Geometry: see drawing. Coordinates: mm, zero at the bounding-box minimum. Coordinates: 2 decimals unless noted, no trailing zeros. Loops run counter-clockwise (first coordinate to the right, second up) from the corner with the lowest first, then second, coordinate; pieces in that order, holes last. Notation, with made-up numbers: (-13.75, -1.75) -> (29.25, -1.75) arc R30 ccw to (29.25, 36.25) -> close; hole circle Ø1 at (-22.5, -38.5). An arc over 180 degrees is marked (long way). Put each result on its own line as item: value. Start each with the question number.
1) Contact query for flat-ended pins moving along their axis: P1, Ø1.5, axis at x = 52.5, z = 1.5, coming from the +Y side; P2, Ø0.9, axis at y = 52.5, z = 1.5, coming from the +X side. Output: stop coordinate, or through.
2) Cut plane C-C (y = 49.5). Return the cut outline in (x, z).
3) Cut plane B-B (x = 49). Return the cut outline in (y, z), plus the area to 3 significant figures.
4) Material intervals for L1, parallel to Y at x = 4.5, z = 2; L2, parallel to Y at x = 10, z = 1.65; L3, parallel to X at y = 48, z = 2.4, sorted ascending.
5) Cut plane A-A (z = 2.5). Return the cut outline in (x, y), plus the area to 3 significant figures.
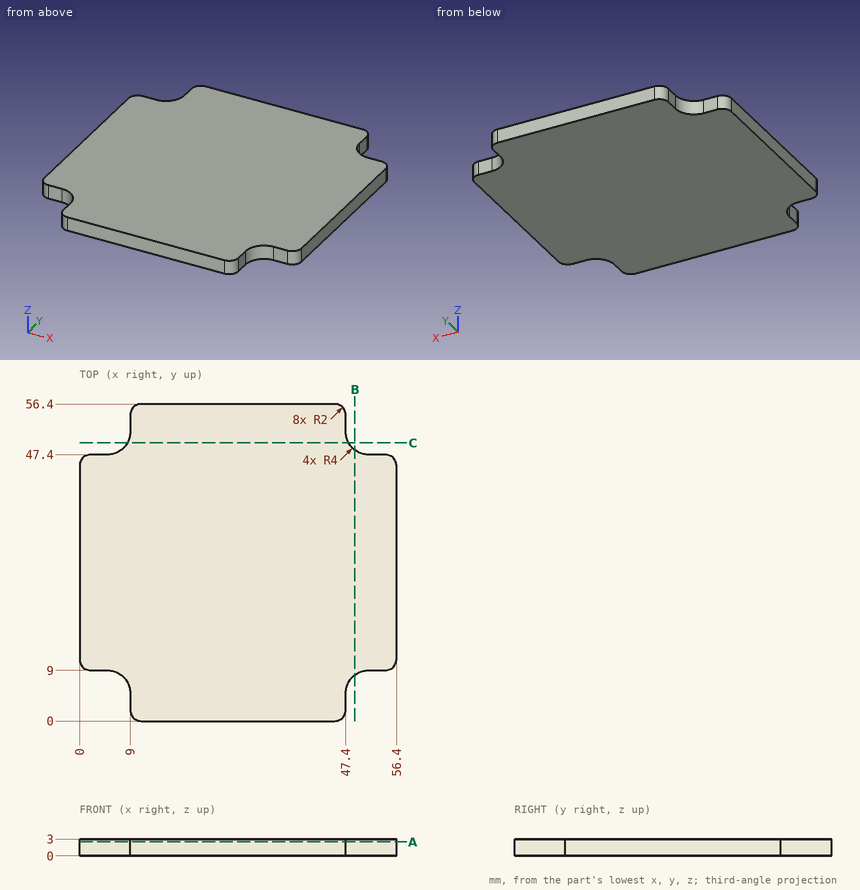
Results found:
1. P1: stops at y = 47.4
1. P2: stops at x = 47.4
2. outline: (8.52, 0) -> (47.88, 0) -> (47.88, 3) -> (8.52, 3) -> close
3. outline: (8.2, 0) -> (48.2, 0) -> (48.2, 3) -> (8.2, 3) -> close
3. area: 120 mm2
4. L1: y = 9 to 47.4
4. L2: y = 0.27 to 56.13
4. L3: x = 7.11 to 49.29
5. outline: (0, 11) arc R2 ccw to (2, 9) -> (5, 9) arc R4 cw to (9, 5) -> (9, 2) arc R2 ccw to (11, 0) -> (45.4, 0) arc R2 ccw to (47.4, 2) -> (47.4, 5) arc R4 cw to (51.4, 9) -> (54.4, 9) arc R2 ccw to (56.4, 11) -> (56.4, 45.4) arc R2 ccw to (54.4, 47.4) -> (51.4, 47.4) arc R4 cw to (47.4, 51.4) -> (47.4, 54.4) arc R2 ccw to (45.4, 56.4) -> (11, 56.4) arc R2 ccw to (9, 54.4) -> (9, 51.4) arc R4 cw to (5, 47.4) -> (2, 47.4) arc R2 ccw to (0, 45.4) -> close
5. area: 2,860 mm2
